The listing builds one solid part. Answer for the finished solid, in the listing's coordinates (mm). A direction names the side the tool comes from. Coordinates: 2 decimals unless noted, no trailing zeros. Loops run counter-clockwise (first coordinate to the right, second up) from the corner with the lowest first, then second, coordinate; pieces in that order, holes last. Notation, with made-up numbers: (9, 42.25) - (49, 42.25) arc R21 ccw to (49, 68.25) - close; hole circle Ø9 at (89, 20.25). An arc over 180 degrees is marked (long way). Return JSON: item names as keys, results as strings. Group by question number.
1. Section A-A (z = 17.5) is taken. Write down the section's boundary in (x, y).
2. Section B-B (y = 159) is taken. Write down the section's boundary in (x, z), and give its area (3 significant figures).
3. The mould has two halves that part along Y. Classify faces 5 (the face through (-52.255, 7.509, -23.846)), 6 (the face through (70, 0, 0)): pulls with the +Y half, pulls with the -Y half, needs draft (parallel to the pull), parting line crosses it, or undercut.
4. Each of these flat-tipped pins is pushed along its axis until it touches: P1, Ø8, axis at x = 11.5, z = -24.5, coming from the +Y side; P2, Ø2, axis at x = 21.5, y = 146, coming from the -Z side; P3, Ø4, axis at y = 48.5, z = 10.5, coming from the -X side. Where does it stop, or does it pass through?
5. Section D-D (z = -12) is taken. Write down the section's boundary in (x, y).
6. Section C-C (x = 21) is taken. Write down the section's boundary in (y, z).
7. Find the intervals of material crossed by line 1 along X through (y, z) = (32.5, -6); line 2 along Z through (x, y) = (-1.5, 215); line 3 along X through (y, z) = (267.5, -2), in increasing order.
8. Which of the six approach directions +Z, -Z, +X, -X, +Y, -Y give full straight-line access (tool end or side, diameter ignored) to faces 1 (the face through (-35, 8, 24)), 2 (the face through (-70, 0, 0)), 3 (the face through (35, 8, 24)), 4 (the face through (10.513, 179.596, 33.384))?
```python
from build123d import *
from build123d.topology import SkipClean

# Parameters (mm, degrees)
SKETCH1_R                = 35
BOSS_EXTRUDE1_DEPTH      = 400
BOSS_EXTRUDE2_DEPTH      = 35
BOSS_EXTRUDE2_DEPTH_BACK = 35
SKETCH3_R                = 35
SKETCH4_R                = 25
BOSS_EXTRUDE3_DEPTH      = 35


with BuildPart() as part:
    # Sketch1 → Boss-Extrude1 (new body)
    with BuildSketch(Plane(origin=(0, 0, 0), x_dir=(1, 0, 0), z_dir=(0, 1, 0))):
        with Locations(Location((0, 0, 0), (0, 0, 270))):
            Circle(SKETCH1_R)
    extrude(amount=BOSS_EXTRUDE1_DEPTH)

    # Sketch2 → Revolve1 (revolve)
    with BuildSketch(Plane(origin=(0, 400, 0), x_dir=(1, 0, 0), z_dir=(0, 1, 0))):
        with BuildLine():
            Line((0, 50), (0, -50))
            ThreePointArc((0, -50), (50, 0), (0, 50))
        make_face()
    revolve(axis=Axis((0, 400, -50), (0, 0, 1)))

    # Sketch3 → Boss-Extrude2 (add, two sides: drawn at the far end of the back side and taken through both)
    with SkipClean():  # the faces are left unmerged after this step: merging them gives an invalid solid
        with BuildSketch(Plane(origin=(0, 0, 0), x_dir=(0, 0, -1), z_dir=(1, 0, 0)).offset(-BOSS_EXTRUDE2_DEPTH_BACK)):
            Circle(SKETCH3_R)
        extrude(amount=BOSS_EXTRUDE2_DEPTH + BOSS_EXTRUDE2_DEPTH_BACK)
    add(part.part.scale(1), mode=Mode.REPLACE)  # the faces are merged on a copy

    # Sketch4 → Boss-Extrude3 (add)
    with SkipClean():  # the faces are left unmerged after this step: merging them gives an invalid solid
        with BuildSketch(Plane(origin=(35, 0, 0), x_dir=(0, 0, -1), z_dir=(1, 0, 0))):
            Circle(SKETCH4_R)
        boss_extrude3 = extrude(amount=BOSS_EXTRUDE3_DEPTH)

    # Mirror1: Boss-Extrude3 across plane
    with SkipClean():  # the faces are left unmerged after this step: merging them gives an invalid solid
        add(boss_extrude3.mirror(Plane(origin=(0, 0, 0), x_dir=(0, 0, 1), z_dir=(1, 0, 0))))


solid = part.part
```
The answers:
{
 "1": {"outline": "(-70, -17.85) - (-35, -17.85) - (-35, -30.31) - (35, -30.31) - (35, -17.85) - (70, -17.85) - (70, 17.85) - (35, 17.85) - (35, 30.31) - (30.31, 30.31) - (30.31, 364.29) arc R46.84 ccw (long way) to (-30.31, 364.29) - (-30.31, 30.31) - (-35, 30.31) - (-35, 17.85) - (-70, 17.85) - close"},
 "2": {"outline": "circle Ø70 at (0, 0)", "area": "3,850 mm2"},
 "3": {"face 5": "undercut", "face 6": "needs draft"},
 "4": {"P1": "stops at y = 444.36", "P2": "stops at z = -28.37", "P3": "stops at x = -33.95"},
 "5": {"outline": "(-70, -21.93) - (-35, -21.93) - (-35, -32.88) - (35, -32.88) - (35, -21.93) - (70, -21.93) - (70, 21.93) - (35, 21.93) - (35, 32.88) - (32.88, 32.88) - (32.88, 364.29) arc R48.54 ccw (long way) to (-32.88, 364.29) - (-32.88, 32.88) - (-35, 32.88) - (-35, 21.93) - (-70, 21.93) - close"},
 "6": {"outline": "(21, -28) - (364.29, -28) arc R45.38 ccw (long way) to (364.29, 28) - (21, 28) arc R35 ccw (long way) to start"},
 "7": {"line 1": "x = -35 to 35", "line 2": "z = -34.97 to 34.97", "line 3": "x = -34.94 to 34.94"},
 "8": {"face 1": "-X", "face 2": "+Z, -Z, -X, +Y, -Y", "face 3": "+X", "face 4": "none"}
}
